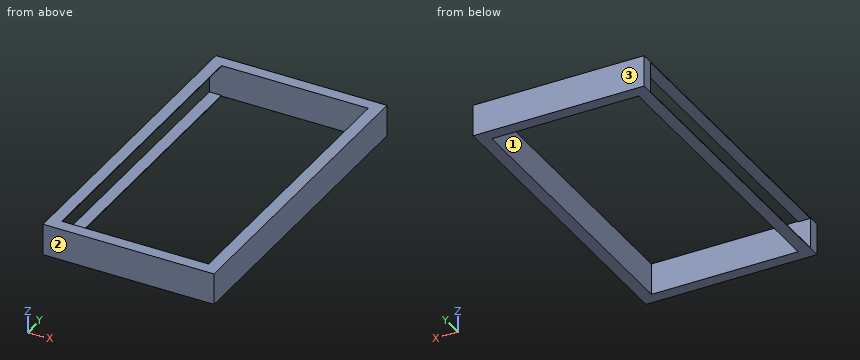
from build123d import *

# Parameters (mm, degrees)
SKETCH2_W           = 261
SKETCH2_H           = 141
SKETCH2_W_2         = 241
SKETCH2_H_2         = 121
BOSS_EXTRUDE1_DEPTH = 26
SKETCH4_W           = 241
SKETCH4_H           = 25
CUT_EXTRUDE1_DEPTH  = 187.727742984


with BuildPart() as part:
    # Sketch2 → Boss-Extrude1 (new body)
    with BuildSketch(Plane(origin=(0, 0, 0), x_dir=(0, 1, 0), z_dir=(0, 0, 1))):
        Rectangle(SKETCH2_W, SKETCH2_H)
        Rectangle(SKETCH2_W_2, SKETCH2_H_2, mode=Mode.SUBTRACT)
    extrude(amount=BOSS_EXTRUDE1_DEPTH)

    # Sketch4 → Cut-Extrude1 (cut, through all)
    with BuildSketch(Plane.YZ.offset(-60.5)):
        with Locations((0, 13)):
            Rectangle(SKETCH4_W, SKETCH4_H)
    extrude(amount=-CUT_EXTRUDE1_DEPTH, mode=Mode.SUBTRACT)


solid = part.part
Geometry check sheet. Reference: the model listing, model coordinates, mm. Face numbers are marked on the shaded views. Give positions to 0.01 mm unless a question says otherwise; leave off trailing zeros. Order: outer loops, then holes, each group sorted by start corner. A loop starts at its lowest first (then second) coordinate and runs counter-clockwise, first axis right, second up. Notation, with made-up numbers: (89.5, 8.5) - (110.5, 8.5) arc R16 ccw to (110.5, 14.5) - close; hole circle Ø2 at (-31.5, -24). An arc over 180 degrees is marked (long way). Use one line per item in the form item = value.
1) Sectioned sample at B-B (y = -31). Record the boundary of the cut face in (x, z).
Working result:
outline = (-70.5, 0) - (-60.5, 0) - (-60.5, 0.5) - (-70.5, 0.5) - close; (-70.5, 25.5) - (-60.5, 25.5) - (-60.5, 26) - (-70.5, 26) - close; (60.5, 0) - (70.5, 0) - (70.5, 26) - (60.5, 26) - close
2) Material ranges on probe 1 along Y at (x, z) = (35, 9); probe 2 along X at (y, z) = (104, 19), recorded low to high. Write a range as from..to.
Working result:
probe_1 = -130.5..-120.5, 120.5..130.5
probe_2 = 60.5..70.5
3) Depth check by flat-ended pin: pin 1 Ø12 at (y, z) = (-14.5, 20) entering from -X; pin 2 Ø8 at (y, z) = (59.5, 15.5) entering from -X. Enter the tip coordinate at first touch or a pass-through.
Working result:
pin_1 = -70.5
pin_2 = 60.5
4) Draft check along Y on the marked faces 1, 2 and 3. Enter one of: released by +Y, released by -Y, zero draft, split by the parting line, or undercut.
Working result:
face_1 = undercut
face_2 = released by -Y
face_3 = released by +Y
5) Sectioned sample at C-C (z = 14). Record the boundary of the cut face in (x, y), and give its area (3 significant figures).
Working result:
outline = (-70.5, -130.5) - (70.5, -130.5) - (70.5, 130.5) - (-70.5, 130.5) - (-70.5, 120.5) - (60.5, 120.5) - (60.5, -120.5) - (-70.5, -120.5) - close
area = 5,230 mm^2
6) Sectioned sample at A-A (x = 50). Record the boundary of the cut face in (y, z), and give its area (3 significant figures).
Working result:
outline = (-130.5, 0) - (-120.5, 0) - (-120.5, 26) - (-130.5, 26) - close; (120.5, 0) - (130.5, 0) - (130.5, 26) - (120.5, 26) - close
area = 520 mm^2
